The model under review builds one solid part; all positions refer to its coordinate system, in mm. Face numbers are marked on the shaded views. A direction names the side the tool comes from. Coordinates: 2 decimals unless noted, no trailing zeros. Order: outer loops, then holes, each group sorted by start corner. A loop starts at its lowest first (then second) coordinate and runs counter-clockwise, first axis right, second up. Notation, with made-up numbers: M 46.5,-29.5 L 93.5,-29.5 A15 cw 93.5,-2.5 Z; hole C -36.5,0.5 d9. An arc over 180 degrees is marked long. Answer as CSV lines item,"result". Start each with the question number.
Q1. Consider section B-B on x = 142.5. Write out the cut boundary in (y, z), and give its area (3 significant figures).
Q2. Wall thickness on L1, parallel to X at y = -174, z = -695; L2, parallel to Z at x = -337, y = 157: over which ranges is each line inside the solid? List them lowest first. Write a range as [from, to].
Q3. Consider section D-D on x = -485. Write out the cut boundary in (y, z) (3 decimals), and give its area (3 significant figures).
Q4. Consider section A-A on z = -342.5. State how many separate pieces and enclosed holes the cut face has, and give its area (3 significant figures).
Q5. For P1, Ø3, axis at x = 443, z = -257.5, coming from the -Y side; P2, Ø2, axis at y = -49.5, z = -201, coming from the +X side; P3, Ø2, axis at x = 36, y = -140.5, coming from the -Z side, all flat-tipped, find the tip position at first contact; note any pin that passes through.
Q6. Machinability: for the marked faces 1, 2, 3, 4 and 5, which of the approach directions +Z, -Z, +X, -X, +Y, -Y give a long, thin tool a straight path to every point of the face, cutting with its end or side? Answer none if there is none.
from build123d import *

# Parameters (mm, degrees)
F0_W      = 266.7
F0_H      = 19.05
F0_W_2    = 6.35
F0_H_2    = 431.8
F0_W_3    = 482.6
F1_DEPTH  = 19.05
F2_DEPTH  = 742.95
F3_R      = 12.7
F4_DEPTH  = 127
F5_DEPTH  = 127
F6_DEPTH  = 742.95
F7_W      = 482.6
F7_H      = 76.2
F7_W_2    = 266.7
F7_H_2    = 193.675
F7_H_3    = 127
F8_DEPTH  = 25.4
F9_W      = 28.575
F9_H      = 101.6
F10_DEPTH = 1104.901


with BuildPart() as f1:
    # F0 (on Top) → F1 (new body)
    with BuildSketch(Plane.XY):
        Polygon((532.898358, 244.44298), (266.198358, 244.44298), (266.198358, 225.39298), (266.198358, -206.40702), (266.198358, -225.45702), (532.898358, -225.45702), (532.898358, -206.40702), (532.898358, 225.39298), align=None)
        Polygon((266.198358, 263.49298), (247.148358, 263.49298), (247.148358, 244.44298), (247.148358, 225.39298), (259.848358, 225.39298), (266.198358, 225.39298), (266.198358, 244.44298), align=None)
        with Locations((399.548358, 253.96798)):
            Rectangle(F0_W, F0_H)
        Polygon((551.948358, 263.49298), (532.898358, 263.49298), (532.898358, 244.44298), (532.898358, 225.39298), (539.248358, 225.39298), (551.948358, 225.39298), align=None)
        with Locations((263.023358, 9.49298)):
            Rectangle(F0_W_2, F0_H_2)
        with Locations((536.073358, 9.49298)):
            Rectangle(F0_W_2, F0_H_2)
        with Locations((-387.851642, 253.96798)):
            Rectangle(F0_W, F0_H)
        Polygon((-235.451642, 263.49298), (-254.501642, 263.49298), (-254.501642, 244.44298), (-254.501642, 225.39298), (-248.151642, 225.39298), (-235.451642, 225.39298), (-235.451642, 244.44298), align=None)
        with Locations((-387.851642, -234.98202)):
            Rectangle(F0_W, F0_H)
        with Locations((399.548358, -234.98202)):
            Rectangle(F0_W, F0_H)
        Polygon((-521.201642, -225.45702), (-521.201642, -206.40702), (-527.551642, -206.40702), (-540.251642, -206.40702), (-540.251642, -244.50702), (-521.201642, -244.50702), align=None)
        Polygon((-248.151642, -206.40702), (-254.501642, -206.40702), (-254.501642, -225.45702), (-254.501642, -244.50702), (-235.451642, -244.50702), (-235.451642, -225.45702), (-235.451642, -206.40702), align=None)
        Polygon((266.198358, -206.40702), (259.848358, -206.40702), (247.148358, -206.40702), (247.148358, -225.45702), (247.148358, -244.50702), (266.198358, -244.50702), (266.198358, -225.45702), align=None)
        Polygon((539.248358, -206.40702), (532.898358, -206.40702), (532.898358, -225.45702), (532.898358, -244.50702), (551.948358, -244.50702), (551.948358, -206.40702), align=None)
        Polygon((-521.201642, 244.44298), (-521.201642, 263.49298), (-540.251642, 263.49298), (-540.251642, 225.39298), (-527.551642, 225.39298), (-521.201642, 225.39298), align=None)
        with Locations((-524.376642, 9.49298)):
            Rectangle(F0_W_2, F0_H_2)
        with Locations((-251.326642, 9.49298)):
            Rectangle(F0_W_2, F0_H_2)
        Polygon((-254.501642, 244.44298), (-521.201642, 244.44298), (-521.201642, 225.39298), (-521.201642, -206.40702), (-521.201642, -225.45702), (-254.501642, -225.45702), (-254.501642, -206.40702), (-254.501642, 225.39298), align=None)
        Polygon((-540.251642, 225.39298), (-540.251642, 263.49298), (-552.951642, 263.49298), (-552.951642, -257.20702), (564.648358, -257.20702), (564.648358, 263.49298), (551.948358, 263.49298), (551.948358, 225.39298), (539.248358, 225.39298), (539.248358, -206.40702), (551.948358, -206.40702), (551.948358, -244.50702), (532.898358, -244.50702), (266.198358, -244.50702), (247.148358, -244.50702), (-235.451642, -244.50702), (-254.501642, -244.50702), (-521.201642, -244.50702), (-540.251642, -244.50702), (-540.251642, -206.40702), (-527.551642, -206.40702), (-527.551642, 225.39298), align=None)
        with Locations((5.848358, 253.96798)):
            Rectangle(F0_W_3, F0_H)
        Polygon((247.148358, 244.44298), (-235.451642, 244.44298), (-235.451642, 225.39298), (-248.151642, 225.39298), (-248.151642, -206.40702), (-235.451642, -206.40702), (-235.451642, -225.45702), (247.148358, -225.45702), (247.148358, -206.40702), (259.848358, -206.40702), (259.848358, 225.39298), (247.148358, 225.39298), align=None)
        with Locations((5.848358, -234.98202)):
            Rectangle(F0_W_3, F0_H)
    extrude(amount=F1_DEPTH)

    # F0 (on Top) → F2 (join)
    with BuildSketch(Plane.XY):
        Polygon((-248.151642, -206.40702), (-254.501642, -206.40702), (-254.501642, -225.45702), (-254.501642, -244.50702), (-235.451642, -244.50702), (-235.451642, -225.45702), (-235.451642, -206.40702), align=None)
        Polygon((-521.201642, -225.45702), (-521.201642, -206.40702), (-527.551642, -206.40702), (-540.251642, -206.40702), (-540.251642, -244.50702), (-521.201642, -244.50702), align=None)
        with Locations((-524.376642, 9.49298)):
            Rectangle(F0_W_2, F0_H_2)
        with Locations((-251.326642, 9.49298)):
            Rectangle(F0_W_2, F0_H_2)
        Polygon((-521.201642, 244.44298), (-521.201642, 263.49298), (-540.251642, 263.49298), (-540.251642, 225.39298), (-527.551642, 225.39298), (-521.201642, 225.39298), align=None)
        Polygon((-235.451642, 263.49298), (-254.501642, 263.49298), (-254.501642, 244.44298), (-254.501642, 225.39298), (-248.151642, 225.39298), (-235.451642, 225.39298), (-235.451642, 244.44298), align=None)
        Polygon((266.198358, 263.49298), (247.148358, 263.49298), (247.148358, 244.44298), (247.148358, 225.39298), (259.848358, 225.39298), (266.198358, 225.39298), (266.198358, 244.44298), align=None)
        Polygon((551.948358, 263.49298), (532.898358, 263.49298), (532.898358, 244.44298), (532.898358, 225.39298), (539.248358, 225.39298), (551.948358, 225.39298), align=None)
        Polygon((266.198358, -206.40702), (259.848358, -206.40702), (247.148358, -206.40702), (247.148358, -225.45702), (247.148358, -244.50702), (266.198358, -244.50702), (266.198358, -225.45702), align=None)
        Polygon((539.248358, -206.40702), (532.898358, -206.40702), (532.898358, -225.45702), (532.898358, -244.50702), (551.948358, -244.50702), (551.948358, -206.40702), align=None)
        with Locations((536.073358, 9.49298)):
            Rectangle(F0_W_2, F0_H_2)
        with Locations((263.023358, 9.49298)):
            Rectangle(F0_W_2, F0_H_2)
    extrude(amount=-F2_DEPTH)

    # F3
    f3_edges = [f1.edges().sort_by_distance(p)[0] for p in [
        (-552.951642, 3.14298, 19.05),
        (5.848358, -257.20702, 19.05),
        (564.648358, 3.14298, 19.05),
    ]]
    fillet(f3_edges, radius=F3_R)

    # F0 (on Top) → F4 (join)
    with BuildSketch(Plane.XY):
        with Locations((5.848358, 253.96798)):
            Rectangle(F0_W_3, F0_H)
    extrude(amount=-F4_DEPTH)

    # F0 (on Top) → F5 (join)
    with BuildSketch(Plane.XY):
        with Locations((5.848358, -234.98202)):
            Rectangle(F0_W_3, F0_H)
    extrude(amount=-F5_DEPTH)

    # F0 (on Top) → F6 (join, through all)
    with BuildSketch(Plane.XY):
        with Locations((-387.851642, -234.98202)):
            Rectangle(F0_W, F0_H)
        with Locations((399.548358, -234.98202)):
            Rectangle(F0_W, F0_H)
    extrude(amount=-F6_DEPTH)

    # F7 (on face) → F8 (cut)
    with BuildSketch(Plane.XZ.offset(244.50702)):
        with Locations((5.848358, -63.5)):
            Rectangle(F7_W, F7_H)
        with Locations((-387.851642, -376.2375)):
            Rectangle(F7_W_2, F7_H_2)
        with Locations((-387.851642, -190.5)):
            Rectangle(F7_W_2, F7_H_3)
        with Locations((-387.851642, -63.5)):
            Rectangle(F7_W_2, F7_H)
        with Locations((-387.851642, -595.3125)):
            Rectangle(F7_W_2, F7_H_2)
        with Locations((399.548358, -595.3125)):
            Rectangle(F7_W_2, F7_H_2)
        with Locations((399.548358, -376.2375)):
            Rectangle(F7_W_2, F7_H_2)
        with Locations((399.548358, -190.5)):
            Rectangle(F7_W_2, F7_H_3)
        with Locations((399.548358, -63.5)):
            Rectangle(F7_W_2, F7_H)
    extrude(amount=-F8_DEPTH, mode=Mode.SUBTRACT)

    # F9 (on face) → F10 (cut, through all)
    with BuildSketch(Plane.YZ.offset(551.948358)):
        with Locations((249.20548, -692.15)):
            Rectangle(F9_W, F9_H)
    extrude(amount=-F10_DEPTH, mode=Mode.SUBTRACT)


solid = f1.part
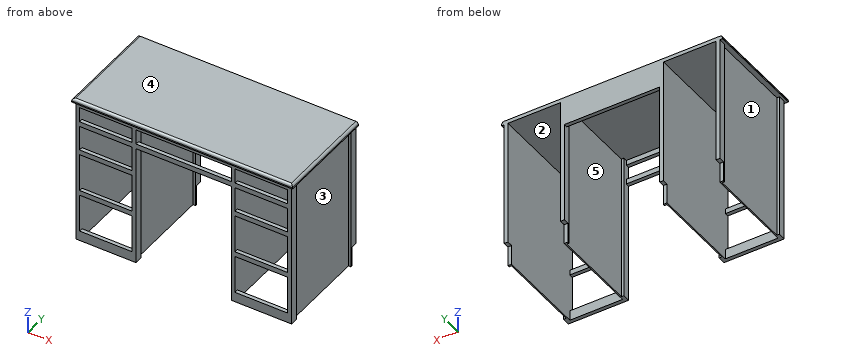
Evaluation:
1,outline,"M -257.21,0 L -244.51,0 L -244.51,-25.4 L -225.46,-25.4 L -225.46,0 L 244.44,0 L 244.44,-127 L 263.49,-127 L 263.49,19.05 L -244.51,19.05 A12.7 ccw -257.21,6.35 Z; M -244.51,-127 L -225.46,-127 L -225.46,-101.6 L -244.51,-101.6 Z"
1,area,"13,300 mm²"
2,L1,"x = [-527.55, -521.2], [-254.5, -248.15], [259.85, 266.2], [532.9, 539.25]"
2,L2,"z = [0, 19.05]"
3,outline,"M -257.207,0 L -244.507,0 L -244.507,-25.4 L -225.457,-25.4 L -225.457,0 L 263.493,0 L 263.493,19.05 L -244.507,19.05 A12.7 ccw -257.207,6.35 Z; M -244.507,-742.95 L -225.457,-742.95 L -225.457,-692.15 L -244.507,-692.15 Z; M -244.507,-498.475 L -225.457,-498.475 L -225.457,-473.075 L -244.507,-473.075 Z; M -244.507,-279.4 L -225.457,-279.4 L -225.457,-254 L -244.507,-254 Z; M -244.507,-127 L -225.457,-127 L -225.457,-101.6 L -244.507,-101.6 Z"
3,area,"12,800 mm²"
4,separate pieces,"4"
4,enclosed holes,"0"
4,area,"16,800 mm²"
5,P1,"stops at y = -244.51"
5,P2,"stops at x = 539.25"
5,P3,"stops at z = 0"
6,face 1,"-Z, -X"
6,face 2,"-Z, +Y"
6,face 3,"-Z, +X"
6,face 4,"+Z, +X, -X, +Y, -Y"
6,face 5,"-Z"
